Autodesk Inventor part; units mm, degrees
ref_plane "YZ Plane" through (0, 0, 0) normal (1, 0, 0) x (0, 1, 0)
ref_plane "XZ Plane" through (0, 0, 0) normal (0, 1, 0) x (-1, 0, 0)
ref_plane "XY Plane" through (0, 0, 0) normal (0, 0, 1) x (1, 0, 0)
sketch "Esboço1" plane through (0, 0, 0) normal (0, 0, 1) x (1, 0, 0)
  line L0 (-13, -24.5) -> (13, -24.5)
  line L1 (13, -24.5) -> (13, 24.5)
  line L2 (13, 24.5) -> (-13, 24.5)
  line L3 (-13, 24.5) -> (-13, -24.5)
  line L4 (-13, -24.5) -> (13, 24.5) construction
  line L5 (13, -24.5) -> (-13, 24.5) construction
  point P0 (0, 0)
  dimension "d0" = 49
  dimension "d1" = 26
extrude "Extrusão1" add sketch "Esboço1" along normal blind 20
sketch "Esboço2" plane through (-13, 24.5, 0) normal (0, 1, 0) x (1, 0, 0)
  circle A0 centre (5, -10) radius 2.5
  line L0 (26, 0) -> (0, 0)
  line L1 (0, 0) -> (0, -20)
  line L2 (26, -20) -> (0, -20)
  line L3 (26, 0) -> (26, -20)
  line L4 (20.5, -14.3301) -> (15.5, -14.3301)
  line L5 (15.5, -14.3301) -> (13, -10)
  line L6 (13, -10) -> (15.5, -5.6699)
  line L7 (15.5, -5.6699) -> (20.5, -5.6699)
  line L8 (20.5, -5.6699) -> (23, -10)
  line L9 (23, -10) -> (20.5, -14.3301)
  circle A1 centre (5, -10) radius 3.5
  line L10 (14.9226, -4.6699) -> (11.8453, -10)
  line L11 (11.8453, -10) -> (14.9226, -15.3301)
  line L12 (14.9226, -15.3301) -> (21.0774, -15.3301)
  line L13 (21.0774, -15.3301) -> (24.1547, -10)
  line L14 (24.1547, -10) -> (21.0774, -4.6699)
  line L15 (21.0774, -4.6699) -> (14.9226, -4.6699)
  point P0 (13, 0)
  point P1 (18, -10)
  dimension "d5" = 5
  dimension "d7" = 5
  dimension "d8" = 5
  dimension "d9" = 13
  dimension "d10" = 10
  dimension "d11" = 10
  dimension "d12" = 5
  dimension "d13" = 1
  dimension "d14" = 1
extrude "Extrusão2" add sketch "Esboço2" along normal blind 1 contours A0 | L4 L5 L6 L7 L8 L9 | A1 | L15 L14 L13 L12 L11 L10
extrude "Extrusão3" cut sketch "Esboço2" against normal blind 1 from surface at 1 contours A0 | L4 L5 L6 L7 L8 L9
fillet "Arredondamento1" radius 1.5 12 edges at (-13, 0, 20) (13, 0, 20) (0, 24.5, 20) (13, 24.5, 10) (-13, 24.5, 10) (0, 24.5, 0) (-13, 0, 0) (-13, -24.5, 10) (0, -24.5, 20) (0, -24.5, 0) (13, -24.5, 10) (13, 0, 0)
properties part number "bateria IC"
Geometry check sheet. Reference: the model listing, model coordinates, mm. A direction names the side the tool comes from. Coordinates: 2 decimals unless noted, no trailing zeros. Loops run counter-clockwise (first coordinate to the right, second up) from the corner with the lowest first, then second, coordinate; pieces in that order, holes last. Notation, with made-up numbers: (65.25, 38) - (77.25, 38) arc R16 ccw to (77.25, 62) - close; hole circle Ø6 at (-18.5, 28.25). An arc over 180 degrees is marked (long way). Use one line per item in the form item = value. Start each with the question number.
Item 1: Section check D-D, the plane x = 9.5. Enter the section's corners in (y, z).
Item 2: Section check C-C, the plane x = -7. Enter the section's corners in (y, z).
Item 3: Tool access check on faces 1 (the face through (5, 25, 15.33)), 2 (the face through (-2, 24.5, 10)), 3 (the face through (9.595, 24.993, 12.702)), 4 (the face through (12.57, 24.05, 10.12)). Record the directions out of +Z, -Z, +X, -X, +Y, -Y that give a thin tool (end or side, any length) a straight path to the whole face; none if there is none.
Item 4: Section check B-B, the plane z = 9.25. Enter the section's corners in (x, y), and give its area (3 significant figures).
Item 5: Section check A-A, the plane x = -3.5. Enter the section's corners in (y, z), and give its area (3 significant figures).
Item 6: Thickness scan on probe 1 along X at (y, z) = (24.8, 10); probe 2 along Z at (x, y) = (-8, 24.9); probe 3 along Y at (x, z) = (-6.5, 15.75). Record the ranges inside material, lowest first.
Item 7: Gauge pin test, flat ends, axial feed: pin 1 (0.8 mm diameter, centred on x = 6, y = 25, fed in from +Z); pin 2 (1.5 mm diameter, centred on x = -7.5, z = 10.5, fed in from +Y). Record the tip position at first contact, or that the pin passes through.
Computed:
q1.outline = (-24.5, 1.5) arc R1.5 ccw to (-23, 0) - (23, 0) arc R1.5 ccw to (24.5, 1.5) - (24.5, 7.13) - (25.5, 7.13) - (25.5, 9.13) - (24.5, 9.13) - (24.5, 10.87) - (25.5, 10.87) - (25.5, 12.87) - (24.5, 12.87) - (24.5, 18.5) arc R1.5 ccw to (23, 20) - (-23, 20) arc R1.5 ccw to (-24.5, 18.5) - close
q2.outline = (-24.5, 1.5) arc R1.5 ccw to (-23, 0) - (23, 0) arc R1.5 ccw to (24.5, 1.5) - (24.5, 6.65) - (25.5, 6.65) - (25.5, 7.71) - (24.5, 7.71) - (24.5, 12.29) - (25.5, 12.29) - (25.5, 13.35) - (24.5, 13.35) - (24.5, 18.5) arc R1.5 ccw to (23, 20) - (-23, 20) arc R1.5 ccw to (-24.5, 18.5) - close
q3.face_1 = +Z, +X, -X, +Y
q3.face_2 = +Y
q3.face_3 = +Z, +X, +Y
q3.face_4 = +Z, -Z, +X, +Y
q4.outline = (-13, -23) arc R1.5 ccw to (-11.5, -24.5) - (11.5, -24.5) arc R1.5 ccw to (13, -23) - (13, 23) arc R1.5 ccw to (11.5, 24.5) - (10.72, 24.5) - (10.72, 25.5) - (9.57, 25.5) - (9.57, 24.5) - (0.43, 24.5) - (0.43, 25.5) - (-0.72, 25.5) - (-0.72, 24.5) - (-4.58, 24.5) - (-4.58, 25.5) - (-5.62, 25.5) - (-5.62, 24.5) - (-10.38, 24.5) - (-10.38, 25.5) - (-11.42, 25.5) - (-11.42, 24.5) - (-11.5, 24.5) arc R1.5 ccw to (-13, 23) - close
q4.area = 1,280 mm2
q5.outline = (-24.5, 1.5) arc R1.5 ccw to (-23, 0) - (23, 0) arc R1.5 ccw to (24.5, 1.5) - (24.5, 18.5) arc R1.5 ccw to (23, 20) - (-23, 20) arc R1.5 ccw to (-24.5, 18.5) - close
q5.area = 978 mm2
q6.probe_1 = -11.5 to -10.5, -5.5 to -4.5, -1.15 to 0, 10 to 11.15
q6.probe_2 = 6.5 to 7.5, 12.5 to 13.5
q6.probe_3 = -24.5 to 24.5
q7.pin_1 = 15.33
q7.pin_2 = 24.5
